```python
from build123d import *

# Parameters (mm, degrees)
ESQUISSE1_W                                  = 80
ESQUISSE1_H                                  = 80
BOSS_EXTRU_1_DEPTH                           = 2
FRAISAGE_POUR_VIS_T_TE_FRAIS_E_BOM_2_COUNT   = 2
FRAISAGE_POUR_VIS_T_TE_FRAIS_E_BOM_2_PITCH   = 65.794986025
FRAISAGE_POUR_VIS_T_TE_FRAIS_E_BOM_3_COUNT   = 2
FRAISAGE_POUR_VIS_T_TE_FRAIS_E_BOM_3_PITCH   = 93.048161572
FRAISAGE_POUR_VIS_T_TE_FRAIS_E_BOM_4_COUNT   = 2
FRAISAGE_POUR_VIS_T_TE_FRAIS_E_BOM_4_PITCH   = 65.794986025
FRAISAGE_POUR_VIS_T_TE_FRAIS_E_BOM_6_A_COUNT = 2
FRAISAGE_POUR_VIS_T_TE_FRAIS_E_BOM_6_A_PITCH = 25.212578074
FRAISAGE_POUR_VIS_T_TE_FRAIS_E_BOM_7_COUNT   = 2
FRAISAGE_POUR_VIS_T_TE_FRAIS_E_BOM_7_PITCH   = 35.655969855
FRAISAGE_POUR_VIS_T_TE_FRAIS_E_BOM_8_COUNT   = 2
FRAISAGE_POUR_VIS_T_TE_FRAIS_E_BOM_8_PITCH   = 25.212578074
CONG_1_R                                     = 1
CONG_2_R                                     = 1


with BuildPart() as part:
    # Esquisse1 → Boss.-Extru.1 (new body)
    with BuildSketch(Plane(origin=(0, 0, 0), x_dir=(1, 0, 0), z_dir=(0, 1, 0))):
        Rectangle(ESQUISSE1_W, ESQUISSE1_H)
    extrude(amount=BOSS_EXTRU_1_DEPTH)

    # Esquisse3 → Fraisage pour vis _ t_te frais_e bomb_e (revolve, cut)
    with BuildSketch(Plane(origin=(-32.897493012, 2, -32.897493012), x_dir=(0, 0, 1), z_dir=(1, 0, 0))):
        Polygon((0, 0), (0, 2), (1.63195, 2), (1.63195, 1.409834001), (2.8575, 0), align=None)
    fraisage_pour_vis_t_te_frais_e_bomb_e = revolve(axis=Axis((-32.897493012, 8.35, -32.897493012), (0, -1, 0)), mode=Mode.SUBTRACT)

    # Fraisage pour vis _ t_te frais_e bom 2: Fraisage pour vis _ t_te frais_e bomb_e ×2
    with Locations(*[(i * FRAISAGE_POUR_VIS_T_TE_FRAIS_E_BOM_2_PITCH, 0, 0) for i in range(1, FRAISAGE_POUR_VIS_T_TE_FRAIS_E_BOM_2_COUNT)]):
        add(fraisage_pour_vis_t_te_frais_e_bomb_e, mode=Mode.SUBTRACT)

    # Fraisage pour vis _ t_te frais_e bom 3: Fraisage pour vis _ t_te frais_e bomb_e ×2
    with Locations(*[Vector(0.707106781, 0, 0.707106781) * (i * FRAISAGE_POUR_VIS_T_TE_FRAIS_E_BOM_3_PITCH) for i in range(1, FRAISAGE_POUR_VIS_T_TE_FRAIS_E_BOM_3_COUNT)]):
        add(fraisage_pour_vis_t_te_frais_e_bomb_e, mode=Mode.SUBTRACT)

    # Fraisage pour vis _ t_te frais_e bom 4: Fraisage pour vis _ t_te frais_e bomb_e ×2
    with Locations(*[(0, 0, i * FRAISAGE_POUR_VIS_T_TE_FRAIS_E_BOM_4_PITCH) for i in range(1, FRAISAGE_POUR_VIS_T_TE_FRAIS_E_BOM_4_COUNT)]):
        add(fraisage_pour_vis_t_te_frais_e_bomb_e, mode=Mode.SUBTRACT)

    # Esquisse6 → Fraisage pour vis _ t_te frais_e bom 5 (revolve, cut)
    with BuildSketch(Plane(origin=(0, 2, 0), x_dir=(0, 0, 1), z_dir=(1, 0, 0))):
        Polygon((0, 0), (0, 2), (1.63195, 2), (1.63195, 1.409834001), (2.8575, 0), align=None)
    revolve(axis=Axis((0, 8.35, 0), (0, -1, 0)), mode=Mode.SUBTRACT)

    # Esquisse8 → Fraisage pour vis _ t_te frais_e bom 6 (revolve, cut)
    with BuildSketch(Plane(origin=(-12.606289037, 2, -12.606289037), x_dir=(0, 0, 1), z_dir=(1, 0, 0))):
        Polygon((0, 0), (0, 2), (1.63195, 2), (1.63195, 1.409834001), (2.8575, 0), align=None)
    fraisage_pour_vis_t_te_frais_e_bom_6 = revolve(axis=Axis((-12.606289037, 8.35, -12.606289037), (0, -1, 0)), mode=Mode.SUBTRACT)

    # Fraisage pour vis _ t_te frais_e bom 6 a: Fraisage pour vis _ t_te frais_e bom 6 ×2
    with Locations(*[(i * FRAISAGE_POUR_VIS_T_TE_FRAIS_E_BOM_6_A_PITCH, 0, 0) for i in range(1, FRAISAGE_POUR_VIS_T_TE_FRAIS_E_BOM_6_A_COUNT)]):
        add(fraisage_pour_vis_t_te_frais_e_bom_6, mode=Mode.SUBTRACT)

    # Fraisage pour vis _ t_te frais_e bom 7: Fraisage pour vis _ t_te frais_e bom 6 ×2
    with Locations(*[Vector(0.707106781, 0, 0.707106781) * (i * FRAISAGE_POUR_VIS_T_TE_FRAIS_E_BOM_7_PITCH) for i in range(1, FRAISAGE_POUR_VIS_T_TE_FRAIS_E_BOM_7_COUNT)]):
        add(fraisage_pour_vis_t_te_frais_e_bom_6, mode=Mode.SUBTRACT)

    # Fraisage pour vis _ t_te frais_e bom 8: Fraisage pour vis _ t_te frais_e bom 6 ×2
    with Locations(*[(0, 0, i * FRAISAGE_POUR_VIS_T_TE_FRAIS_E_BOM_8_PITCH) for i in range(1, FRAISAGE_POUR_VIS_T_TE_FRAIS_E_BOM_8_COUNT)]):
        add(fraisage_pour_vis_t_te_frais_e_bom_6, mode=Mode.SUBTRACT)

    # Congé1
    cong_1_edges = [part.edges().sort_by_distance(p)[0] for p in [
        (-40, 1, 40),
    ]]
    fillet(cong_1_edges, radius=CONG_1_R)

    # Congé2
    cong_2_edges = [part.edges().sort_by_distance(p)[0] for p in [
        (40, 1, 40),
        (-40, 1, -40),
        (40, 1, -40),
    ]]
    fillet(cong_2_edges, radius=CONG_2_R)


solid = part.part
```
CAD build for the part. Positions are in the model's coordinates, mm. Round coordinates to 2 decimals unless told otherwise and drop trailing zeros. Order: outer loops, then holes, each group sorted by start corner. A loop starts at its lowest first (then second) coordinate and runs counter-clockwise, first axis right, second up.
Item 1: Saw through at C-C on y = 1. State how many separate pieces and enclosed holes the cut face has, then the cut area to 3 significant figures.
Item 2: Pin check, flat tips, straight feed: pin 1 (2 mm diameter, centred on x = -12.61, z = 12.61, fed in from -Y); pin 2 (4 mm diameter, centred on x = 0, z = 0, fed in from +Y); pin 3 (5 mm diameter, centred on x = 32.9, z = 32.9, fed in from +Y). Stop position of each tip, or through.
Item 3: Mould opens along Z. For faces 1 (the face through (8, 0, -1)), 2 (the face through (1.593, 0.299, -0.354)), 3 (the face through (-1, 1, 40)) say: pulls with the +Z half, pulls with the -Z half, needs draft (parallel to the pull), parting line crosses it, or undercut.
Item 4: Saw through at A-A on z = 0. Write the cut outline in (x, y).
Item 5: Probe line 1 along Z through (x, y) = (-14, 0.5); line 2 along Z through (x, y) = (-34, 1.8); line 3 along X through (y, z) = (1.1, 12.5). List the from-to ranges inside material, lowest first.
Item 6: Saw through at B-B on x = 0. Write the cut outline in (y, z), then the cut area to 3 significant figures.
Reported:
1. separate pieces: 1
1. enclosed holes: 9
1. area: 6,290 mm2
2. pin 1: passes through
2. pin 2: stops at y = 1.01
2. pin 3: stops at y = 1.59
3. face 1: needs draft
3. face 2: undercut
3. face 3: pulls with the +Z half
4. outline: (-40, 0) - (-1.63, 0) - (-1.63, 0.59) - (-2.86, 2) - (-40, 2) - close; (1.63, 0) - (40, 0) - (40, 2) - (2.86, 2) - (1.63, 0.59) - close
5. line 1: z = -40 to -13.46, -11.76 to 11.76, 13.46 to 40
5. line 2: z = -40 to -35.34, -30.45 to 30.45, 35.34 to 40
5. line 3: x = -40 to -14.68, -10.53 to 10.53, 14.68 to 40
6. outline: (0, -40) - (2, -40) - (2, -2.86) - (0.59, -1.63) - (0, -1.63) - close; (0, 1.63) - (0.59, 1.63) - (2, 2.86) - (2, 40) - (0, 40) - close
6. area: 152 mm2
